Verification items for the finished model (mm, model axes). Round coordinates to 2 decimals unless told otherwise and drop trailing zeros. Order: outer loops, then holes, each group sorted by start corner. A loop starts at its lowest first (then second) coordinate and runs counter-clockwise, first axis right, second up. Notation, with made-up numbers: M -24.75,-25.75 L -12.75,-25.75 A8 cw -12.75,-14.75 Z; hole C 25.5,-14.75 d1. An arc over 180 degrees is marked long. Answer as a JSON object with one key per item and string values. Group by question number.
```python
from build123d import *

# Parameters (mm, degrees)
F1_DEPTH = 25.4
F3_DEPTH = 3.175


with BuildPart() as f1:
    # F0 (on Right) → F1 (new body)
    with BuildSketch(Plane.YZ):
        with BuildLine():
            Line((-71.363949, 338.589144), (-357.113949, 338.589144))
            Line((-357.113949, 338.589144), (-357.113949, -64.635856))
            Line((-357.113949, -64.635856), (-341.238949, -64.635856))
            ThreePointArc((-341.238949, -64.635856), (-214.238949, 52.839144), (-87.238949, -64.635856))
            Line((-87.238949, -64.635856), (-71.363949, -64.635856))
            Line((-71.363949, -64.635856), (-71.363949, 338.589144))
        make_face()
    extrude(amount=F1_DEPTH)

    # F2 (on face) → F3 (cut)
    with BuildSketch(Plane.YZ.offset(25.4)):
        with BuildLine():
            Line((-204.713949, 338.589144), (-214.238949, 338.589144))
            Line((-214.238949, 338.589144), (-223.763949, 338.589144))
            Line((-223.763949, 338.589144), (-223.763949, 52.48254))
            ThreePointArc((-223.763949, 52.48254), (-214.238949, 52.839144), (-204.713949, 52.48254))
            Line((-204.713949, 52.48254), (-204.713949, 338.589144))
        make_face()
        with BuildLine():
            ThreePointArc((-204.713949, 52.48254), (-214.238949, 52.839144), (-223.763949, 52.48254))
            Line((-223.763949, 52.48254), (-223.763949, 26.907945))
            Line((-223.763949, 26.907945), (-204.713949, 26.907945))
            Line((-204.713949, 26.907945), (-204.713949, 52.48254))
        make_face()
    extrude(amount=-F3_DEPTH, mode=Mode.SUBTRACT)


solid = f1.part
```
Q1. Cross-section at A-A, the plane z = 1. Record the cut outline in (x, y).
Q2. Release check for a two-part mould opening along Y. For faces 1 (the face through (22.225, -214, 198)), 2 (the face through (13, -357.114, 140)), 3 (the face through (12.52, -216.9, 52.81)), 4 (the face through (13, -79, -64.636)) record: released by +Y, released by -Y, zero draft, split by the parting line, or undercut.
Q3. Gauge pin test, flat ends, axial feed: pin 1 Ø6 at (x, y) = (10.5, -294.5) entering from -Z; pin 2 Ø21 at (y, z) = (-209.5, 249.5) entering from +X; pin 3 Ø6 at (x, y) = (12.5, -153.5) entering from -Z. Record the tip position at first contact, or that the pin passes through.
Q4. Cross-section at D-D, the plane y = -94. Record the cut outline in (x, z), then the cut area to 3 significant figures.
Q5. Cross-section at B-B, the plane x = 17.75. Record the cut outline in (y, z).
Q6. Cross-section at C-C, the plane z = 45. Record the cut outline in (x, y), then the cut area to 3 significant figures.
Q7. Thickness scan on line 1 (Y direction, x = 23, z = 137); line 2 (Z direction, x = 21, y = -297); line 3 (Y direction, x = 11, z = -26). Record the ranges inside material, lowest first. Write a range as from..to.
Conclusion:
{
 "1": {"outline": "M 0,-357.11 L 25.4,-357.11 L 25.4,-316.81 L 0,-316.81 Z; M 0,-111.67 L 25.4,-111.67 L 25.4,-71.36 L 0,-71.36 Z"},
 "2": {"face 1": "undercut", "face 2": "released by -Y", "face 3": "undercut", "face 4": "zero draft"},
 "3": {"pin 1": "z = 21.86", "pin 2": "x = 25.4", "pin 3": "z = 35.75"},
 "4": {"outline": "M 0,-32.48 L 25.4,-32.48 L 25.4,338.59 L 0,338.59 Z", "area": "9,430 mm2"},
 "5": {"outline": "M -357.11,-64.64 L -341.24,-64.64 A127.39 cw -87.24,-64.64 L -71.36,-64.64 L -71.36,338.59 L -357.11,338.59 Z"},
 "6": {"outline": "M 0,-357.11 L 25.4,-357.11 L 25.4,-258.24 L 0,-258.24 Z; M 0,-170.24 L 25.4,-170.24 L 25.4,-71.36 L 0,-71.36 Z", "area": "5,020 mm2"},
 "7": {"line 1": "-357.11..-223.76, -204.71..-71.36", "line 2": "22.29..338.59", "line 3": "-357.11..-332.01, -96.47..-71.36"}
}
